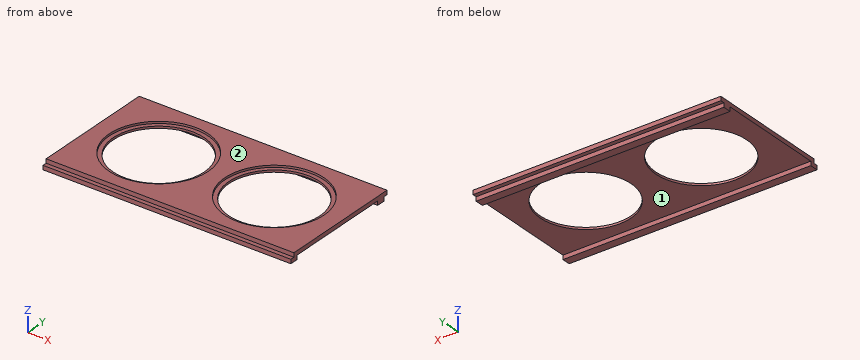
```python
from build123d import *

# Parameters (mm, degrees)
F0_W     = 600
F0_H     = 300
F0_R     = 120
F1_DEPTH = 10
F0_R_2   = 110
F2_DEPTH = 5
F3_W     = 600
F3_H     = 10
F4_DEPTH = 10


with BuildPart() as f1:
    # F0 (on Top) → F1 (new body)
    with BuildSketch(Plane.XY):
        Rectangle(F0_W, F0_H)
        with Locations((-140, 0)):
            Circle(F0_R, mode=Mode.SUBTRACT)
        with Locations((140, 0)):
            Circle(F0_R, mode=Mode.SUBTRACT)
    extrude(amount=F1_DEPTH)

    # F0 (on Top) → F2 (join)
    with BuildSketch(Plane.XY):
        with Locations((-140, 0)):
            Circle(F0_R)
        with Locations((-140, 0)):
            Circle(F0_R_2, mode=Mode.SUBTRACT)
        with Locations((140, 0)):
            Circle(F0_R)
        with Locations((140, 0)):
            Circle(F0_R_2, mode=Mode.SUBTRACT)
    extrude(amount=F2_DEPTH)

    # F3 (on face) → F4 (join)
    with BuildSketch(Plane.XY):
        with Locations((0, -145)):
            Rectangle(F3_W, F3_H)
        with Locations((0, -155)):
            Rectangle(F3_W, F3_H)
        Polygon((300, 140), (-300, 140), (-300, 120), (-140, 120), (140, 120), (300, 120), align=None)
    extrude(amount=-F4_DEPTH)


solid = f1.part
```
CAD build for the part. Positions are in the model's coordinates, mm. Face numbers are marked on the shaded views. Coordinates: 2 decimals unless noted, no trailing zeros. Loops run counter-clockwise (first coordinate to the right, second up) from the corner with the lowest first, then second, coordinate; pieces in that order, holes last. Notation, with made-up numbers: (-13, 62.5) - (45, 62.5) arc R22 ccw to (45, 89.5) - close; hole circle Ø7 at (35.25, -13.75). An arc over 180 degrees is marked (long way). Use CSV: the item, a comma, the result in double quotes. Start each with the question number.
Q1. Cut at D-D, the plane y = -128. List the corners of the cut face in (x, z).
Q2. Cut at A-A, the plane x = -140. List the corners of the cut face in (y, z).
Q3. Probe probe 1 along X at (y, z) = (2.5, 7.5); probe 2 along Y at (x, z) = (140, 2.5); probe 3 along Y at (x, z) = (244, -2.25). List the from-to ranges inside material, lowest first. Write a range as from..to.
Q4. Cut at B-B, the plane y = 0. List the corners of the cut face in (x, z), then the cut area to 3 significant figures.
Q5. Drop flat-ended pins along their axis: P1, Ø11, axis at x = 17, y = -156, coming from the +Z side; P2, Ø8, axis at x = -1.5, z = -7, coming from the +Y side; P3, Ø11, axis at x = -102.5, y = 147, coming from the -Z side. Give the stop position or say it passes through.
Q6. Two-plate mould, pull along Y, no slides. Class the marked faces 1 and 2: +Y half, -Y half, draft (parallel to the pull), parting line (faces both ways), or undercut.
Q7. Cut at C-C, the plane z = -4.5. List the corners of the cut face in (x, y), then the cut area to 3 significant figures.
Here are the results:
1,outline,"(-300, 0) - (300, 0) - (300, 10) - (-300, 10) - close"
2,outline,"(-160, -10) - (-140, -10) - (-140, 0) - (-110, 0) - (-110, 5) - (-120, 5) - (-120, 10) - (-150, 10) - (-150, 0) - (-160, 0) - close; (110, 0) - (120, 0) - (120, -10) - (140, -10) - (140, 0) - (150, 0) - (150, 10) - (120, 10) - (120, 5) - (110, 5) - close"
3,probe 1,"-300..-259.97, -20.03..20.03, 259.97..300"
3,probe 2,"-150..-110, 110..150"
3,probe 3,"-160..-140, 120..140"
4,outline,"(-300, 0) - (-250, 0) - (-250, 5) - (-260, 5) - (-260, 10) - (-300, 10) - close; (-30, 0) - (30, 0) - (30, 5) - (20, 5) - (20, 10) - (-20, 10) - (-20, 5) - (-30, 5) - close; (250, 0) - (300, 0) - (300, 10) - (260, 10) - (260, 5) - (250, 5) - close"
4,area,"1,400 mm2"
5,P1,"z = 0"
5,P2,"y = 140"
5,P3,"z = 0"
6,face 1,"undercut"
6,face 2,"draft"
7,outline,"(-300, -160) - (300, -160) - (300, -140) - (-300, -140) - close; (-300, 120) - (300, 120) - (300, 140) - (-300, 140) - close"
7,area,"24,000 mm2"
